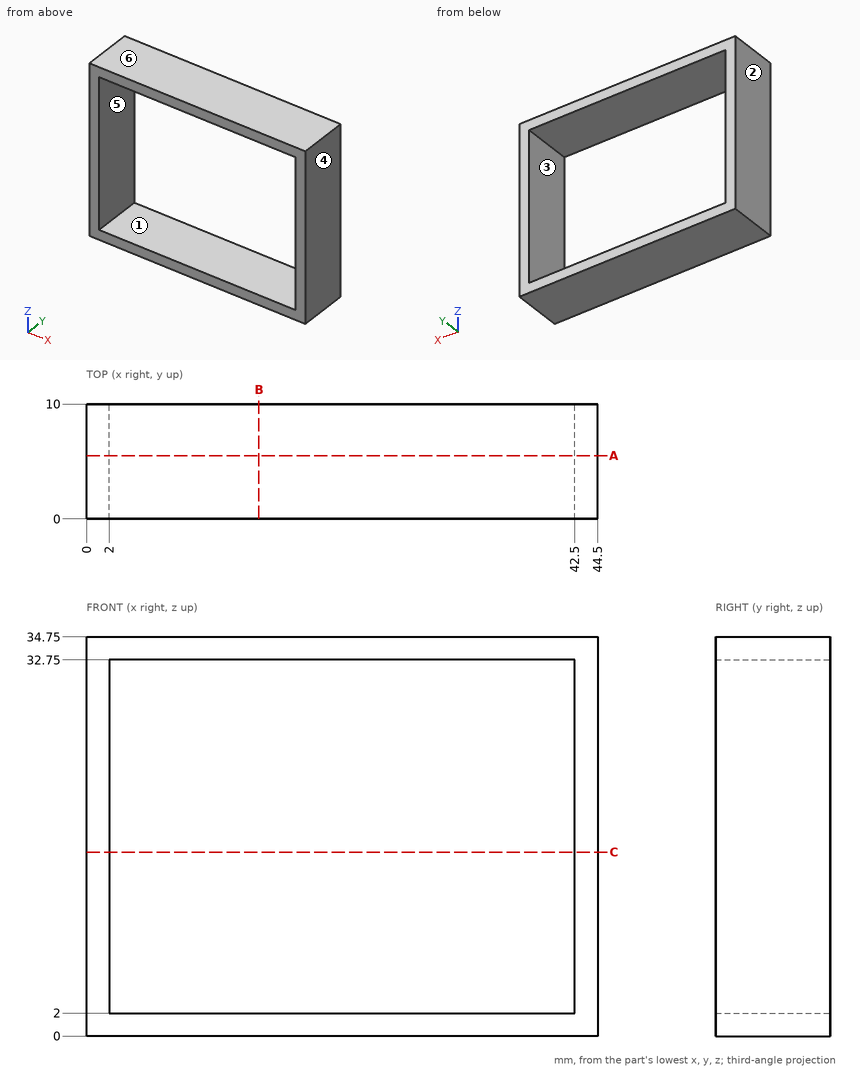
Design review of the part shown in the three views and the two pictorial views. Dimensions are in mm from the part's minimum x, y and z. A direction names the side the tool comes from. Give positions to 0.01 mm unless a question says otherwise; leave off trailing zeros. Write each loop counter-clockwise with the first axis right and the second up, starting at its lowest first coordinate (ties: lowest second). Pieces come first, ordered by that corner, then holes. Notation, with made-up numbers: M 56,36 L 60,36 A15 cw 60,46 Z; hole C 64,-15.5 d9. An arc over 180 degrees is marked long. Return JSON: item names as keys, results as strings. Group by question number.
Item 1: Take a section at A-A (y = 5.5). Give the boundary of the cut face in (x, z).
Item 2: The part is to be moulded in two halves that separate along X. For the marked faces 3, 4, 5 and 6, say which applies: pulls with the +X half, pulls with the -X half, needs draft (parallel to the pull), parting line crosses it, or undercut.
Item 3: Take a section at B-B (x = 15). Give the boundary of the cut face in (y, z).
Item 4: Wall thickness on line 1 along X through (y, z) = (5.5, 11); line 2 along Z through (x, y) = (21, 2.5): over which ranges is each line inside the solid? List them lowest first.
Item 5: Take a section at C-C (z = 16). Give the boundary of the cut face in (x, y), plus the area to 3 significant figures.
Item 6: Tool access review of the marked faces 1 and 2: name each direction out of +Z, -Z, +X, -X, +Y, -Y from which nothing blocks a thin tool from reaching the whole face with its end or side.
Return value:
{
 "1": {"outline": "M 0,0 L 44.5,0 L 44.5,34.75 L 0,34.75 Z; hole M 2,2 L 42.5,2 L 42.5,32.75 L 2,32.75 Z"},
 "2": {"face 3": "undercut", "face 4": "pulls with the +X half", "face 5": "undercut", "face 6": "needs draft"},
 "3": {"outline": "M 0,0 L 10,0 L 10,2 L 0,2 Z; M 0,32.75 L 10,32.75 L 10,34.75 L 0,34.75 Z"},
 "4": {"line 1": "x = 0 to 2, 42.5 to 44.5", "line 2": "z = 0 to 2, 32.75 to 34.75"},
 "5": {"outline": "M 0,0 L 2,0 L 2,10 L 0,10 Z; M 42.5,0 L 44.5,0 L 44.5,10 L 42.5,10 Z", "area": "40.0 mm2"},
 "6": {"face 1": "+Y, -Y", "face 2": "+Z, -Z, -X, +Y, -Y"}
}
